The model under review builds one solid part; all positions refer to its coordinate system, in mm. A direction names the side the tool comes from. Round coordinates to 2 decimals unless told otherwise and drop trailing zeros. Write each loop counter-clockwise with the first axis right and the second up, starting at its lowest first coordinate (ties: lowest second). Pieces come first, ordered by that corner, then holes. Notation, with made-up numbers: (32, 10) - (60, 10) arc R18 cw to (60, 15) - close; hole circle Ø4 at (32.5, 33.5). An arc over 180 degrees is marked (long way). Write each question's results on one line, items separated by ' | '.
Autodesk Inventor part; units mm, degrees
ref_plane "YZ Plane" through (0, 0, 0) normal (1, 0, 0) x (0, 1, 0)
ref_plane "XZ Plane" through (0, 0, 0) normal (0, 1, 0) x (-1, 0, 0)
ref_plane "XY Plane" through (0, 0, 0) normal (0, 0, 1) x (1, 0, 0)
sketch "Szkic1" plane through (0, 0, 0) normal (0, 1, 0) x (-1, 0, 0)
  line L0 (0, 0) -> (300, 0)
  line L1 (300, 0) -> (300, -100)
  line L2 (300, -100) -> (0, -100)
  line L3 (0, -100) -> (0, 0)
  dimension "d0" = 100
  dimension "d1" = 300
sketch "Szkic2" plane through (0, 0, 0) normal (0, 1, 0) x (-1, 0, 0)
  line L0 (15, -15) -> (285, -15)
  line L1 (285, -15) -> (285, -85)
  line L2 (285, -85) -> (15, -85)
  line L3 (15, -85) -> (15, -15)
  point P0 (0, 0)
  dimension "d2" = 270
  dimension "d3" = 70
  dimension "d4" = 15
  dimension "d5" = 15
extrude "Wyciągnięcie proste1" add sketch "Szkic1" along normal blind 15
extrude "Wyciągnięcie proste2" cut sketch "Szkic2" along normal blind 15
fillet "Zaokrąglenie1" radius 2 8 edges at (-285, 7.5, -85) (-15, 7.5, -85) (-15, 7.5, -15) (-285, 7.5, -15) (-300, 7.5, 0) (-300, 7.5, -100) (0, 7.5, -100) (0, 7.5, 0)
sketch "Szkic3" plane through (0, 15, 0) normal (0, 1, 0) x (1, 0, 0)
  line L0 (0, 2) -> (0, 98)
  line L1 (-2, 100) -> (-298, 100)
  line L2 (-298, 0) -> (-2, 0)
  line L3 (-300, 98) -> (-300, 2)
  point P0 (0, 0)
  point P1 (-5, 86)
  point P2 (-5, 14)
  point P3 (-295, 86)
  point P4 (-295, 14)
  dimension "d11" = 5
  dimension "d12" = 14
  dimension "d13" = 14
  dimension "d14" = 14
  dimension "d15" = 5
  dimension "d16" = 5
  dimension "d17" = 5
  dimension "d18" = 14
hole "Otwór1" at (-5, 15, -86) at (-5, 15, -14) at (-295, 15, -86) at (-295, 15, -14) direction (0, -1, 0) diameter 5 depth 15
sketch "Szkic4" plane through (0, 15, 0) normal (0, 1, 0) x (1, 0, 0)
  point P0 (0, 0)
sketch "Szkic5" plane through (0, 0, -2) normal (1, 0, 0) x (0, 0, -1)
  line L0 (55.525, 13.5) -> (62.525, 13.5)
  line L1 (62.525, 13.5) -> (62.525, 13)
  line L2 (62.525, 13) -> (55.525, 13)
  line L3 (55.525, 13) -> (55.525, 13.5)
  line L4 (0, 15) -> (96, 15)
  line L5 (98, 0) -> (98, 15)
  point P0 (-2, 0)
  point P1 (62.525, 13.25)
  dimension "d26" = 7
  dimension "d27" = 0.5
  dimension "d28" = 1.5
  dimension "d29" = 35.475
extrude "Wyciągnięcie proste3" cut sketch "Szkic5" against normal through all
properties part number "podstawka_prowadzaca"
Q1. Insertion check: P1, Ø3, axis at x = -295, z = -86, coming from the +Y side; P2, Ø6, axis at x = -295, z = -14, coming from the -Y side. Each pin has a flat end and moves straight along its axis. Give the tip position at first contact, or say it passes through.
Evaluation:
P1: passes through | P2: stops at y = 0
Q2. For probe 1 along Z at (x, y) = (-295, 10); probe 2 along X at (y, z) = (8.75, -14); probe 3 along X at (y, z) = (8.5, -53.5), list the stretches that pass through material, from the lowest coordinate up.
Evaluation:
probe 1: z = -100 to -88.5, -83.5 to -16.5, -11.5 to 0 | probe 2: x = -300 to -297.5, -292.5 to -7.5, -2.5 to 0 | probe 3: x = -300 to -285, -15 to 0
Q3. We need section A-A (y = 9.5). State the section outline as (x, z) points.
Evaluation:
outline: (-300, -98) arc R2 ccw to (-298, -100) - (-2, -100) arc R2 ccw to (0, -98) - (0, -2) arc R2 ccw to (-2, 0) - (-298, 0) arc R2 ccw to (-300, -2) - close; hole circle Ø5 at (-295, -86); hole circle Ø5 at (-295, -14); hole (-285, -83) arc R2 ccw to (-283, -85) - (-17, -85) arc R2 ccw to (-15, -83) - (-15, -17) arc R2 ccw to (-17, -15) - (-283, -15) arc R2 ccw to (-285, -17) - close; hole circle Ø5 at (-5, -86); hole circle Ø5 at (-5, -14)
Q4. Tool access review of faces 1 (the flat face through (-7, 13.5, -61)), 2 (the flat face through (-285, 7, -50)), 3 (the flat face through (-149, 15, -91)): name each direction out of +Z, -Z, +X, -X, +Y, -Y from which nothing blocks a thin tool from reaching the whole face with its end or side.
Evaluation:
face 1: +X, -X | face 2: +Y, -Y | face 3: +Z, -Z, +X, -X, +Y
Q5. We need section B-B (x = -220). State the section outline as (y, z) points.
Evaluation:
outline: (0, -100) - (15, -100) - (15, -85) - (0, -85) - close; (0, -15) - (15, -15) - (15, 0) - (0, 0) - close
Q6. The part is to be moulded in two halves that separate along X. For faces 4 (the flat face through (-7, 13, -61)), 5 (the flat face through (-148, 7, -15)), 6 (the cylindrical face through (-6.69, 7.4, -15.84)), 7 (the flat face through (-300, 7, -49)), say which applies: released by +X, released by -X, zero draft, split by the parting line, or undercut.
Evaluation:
face 4: zero draft | face 5: undercut | face 6: undercut | face 7: released by -X
Q7. We need section C-C (z = -74.5). State the section outline as (x, y) points.
Evaluation:
outline: (-300, 0) - (-285, 0) - (-285, 15) - (-300, 15) - close; (-15, 0) - (0, 0) - (0, 15) - (-15, 15) - close
